Input: part model. Units: mm. Frame: model coordinates. Face numbers are marked on the shaded views. Give positions to 0.01 mm unless a question says otherwise; leave off trailing zeros. Answer as CSV lines item,"result".
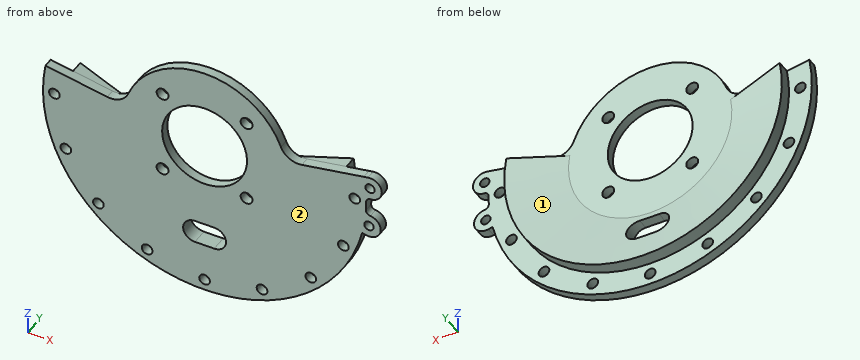
```python
from build123d import *

# Parameters (mm, degrees)
SKETCH1_R           = 1.8
SKETCH1_R_2         = 2
SKETCH1_R_3         = 14.2875
BOSS_EXTRUDE1_DEPTH = 3.175
REVOLVE3_ANGLE      = 200
BOSS_EXTRUDE2_START = -3.175
SKETCH3_R           = 1.5875
BOSS_EXTRUDE2_DEPTH = 3.175
CUT_EXTRUDE1_DEPTH  = 81.857095427


# Read off the part's stored shape, not the designer's step: Revolve3
with BuildPart() as part:
    # Sketch1 → Boss-Extrude1 (new body)
    with BuildSketch(Plane(origin=(0, 0, 0), x_dir=(1, 0, 0), z_dir=(0, 1, 0))):
        with BuildLine():
            Line((53.576531883, -9.446988104), (32.743932203, -5.773638702))
            ThreePointArc((32.743932203, -5.773638702), (28.505328465, -6.505538278), (25.705607757, -9.770963609))
            ThreePointArc((25.705607757, -9.770963609), (0, -27.5), (-25.705607757, -9.770963609))
            ThreePointArc((-25.705607757, -9.770963609), (-28.505328465, -6.505538278), (-32.743932203, -5.773638702))
            Line((-32.743932203, -5.773638702), (-53.576531883, -9.446988104))
            ThreePointArc((-53.576531883, -9.446988104), (0, 54.403036246), (53.576531883, -9.446988104))
        make_face()
        with Locations(Location((-50.569518123, 0, 0), (0, 0, 270))):
            Circle(SKETCH1_R, mode=Mode.SUBTRACT)
        with Locations(Location((-46.720142763, 19.352116768, 0), (0, 0, 270))):
            Circle(SKETCH1_R, mode=Mode.SUBTRACT)
        with Locations(Location((-35.758049186, 35.758049186, 0), (0, 0, 270))):
            Circle(SKETCH1_R, mode=Mode.SUBTRACT)
        with Locations(Location((-19.352116768, 46.720142763, 0), (0, 0, 270))):
            Circle(SKETCH1_R, mode=Mode.SUBTRACT)
        with Locations(Location((0, 50.569518123, 0), (0, 0, 270))):
            Circle(SKETCH1_R, mode=Mode.SUBTRACT)
        with Locations(Location((19.352116768, 46.720142763, 0), (0, 0, 270))):
            Circle(SKETCH1_R, mode=Mode.SUBTRACT)
        with Locations(Location((35.758049186, 35.758049186, 0), (0, 0, 270))):
            Circle(SKETCH1_R, mode=Mode.SUBTRACT)
        with Locations(Location((46.720142763, 19.352116768, 0), (0, 0, 270))):
            Circle(SKETCH1_R, mode=Mode.SUBTRACT)
        with Locations(Location((50.569518123, 0, 0), (0, 0, 270))):
            Circle(SKETCH1_R, mode=Mode.SUBTRACT)
        with Locations(Location((14.142135624, 14.142135624, 0), (0, 0, 270))):
            Circle(SKETCH1_R_2, mode=Mode.SUBTRACT)
        with Locations(Location((-14.142135624, 14.142135624, 0), (0, 0, 270))):
            Circle(SKETCH1_R_2, mode=Mode.SUBTRACT)
        with Locations(Location((-14.142135624, -14.142135624, 0), (0, 0, 270))):
            Circle(SKETCH1_R_2, mode=Mode.SUBTRACT)
        with Locations(Location((14.142135624, -14.142135624, 0), (0, 0, 270))):
            Circle(SKETCH1_R_2, mode=Mode.SUBTRACT)
        with Locations(Location((0, 0, 0), (0, 0, 270))):
            Circle(SKETCH1_R_3, mode=Mode.SUBTRACT)
        with BuildLine():
            Line((-3.25, 37.54875), (3.25, 37.54875))
            ThreePointArc((3.25, 37.54875), (7.21875, 33.58), (3.25, 29.61125))
            Line((3.25, 29.61125), (-3.25, 29.61125))
            ThreePointArc((-3.25, 29.61125), (-7.21875, 33.58), (-3.25, 37.54875))
        make_face(mode=Mode.SUBTRACT)
    extrude(amount=-BOSS_EXTRUDE1_DEPTH)

    # Revolve3 outline → Revolve3 (revolve)
    with BuildSketch(Plane(origin=(0, 0, 0), x_dir=(0.9848077530122042, 0, 0.1736481776669518), z_dir=(-0.1736481776669518, 0, 0.9848077530122042))):
        Polygon((46.736, 0), (46.736, 4.35512275), (27.5, 0), align=None)
    revolve(axis=Axis((0, 0, 0), (0, 1, 0)), revolution_arc=REVOLVE3_ANGLE)

    # Sketch3 → Boss-Extrude2 (add)
    with BuildSketch(Plane.XZ.offset(3.175).offset(BOSS_EXTRUDE2_START)):
        with BuildLine():
            Line((53.060117126, -12.013089669), (54.471072105, -12.3325373))
            ThreePointArc((54.471072105, -12.3325373), (59.259341774, -9.131069871), (55.807809409, -4.519796246))
            ThreePointArc((55.807809409, -4.519796246), (54.72616849, -3.989558211), (54.328198384, -2.85258009))
            ThreePointArc((54.328198384, -2.85258009), (54.387291369, -1.308774374), (54.402523984, 0.236086798))
            ThreePointArc((54.402523984, 0.236086798), (54.854722203, 1.352606489), (55.960615645, 1.830203754))
            ThreePointArc((55.960615645, 1.830203754), (59.629955631, 6.270120891), (55.001219172, 9.698198912))
            Line((55.001219172, 9.698198912), (53.576531883, 9.446988104))
            Line((53.576531883, 9.446988104), (53.060117126, -12.013089669))
        make_face()
        with Locations(Location((55.690385377, 5.789743142, 0), (0, 0, 270))):
            Circle(SKETCH3_R, mode=Mode.SUBTRACT)
        with Locations(Location((55.347437708, -8.461754447, 0), (0, 0, 270))):
            Circle(SKETCH3_R, mode=Mode.SUBTRACT)
    extrude(amount=BOSS_EXTRUDE2_DEPTH)

    # Sketch4 → Cut-Extrude1 (cut, through all)
    with BuildSketch(Plane.XZ):
        with BuildLine():
            Line((-3.25, -37.54875), (3.25, -37.54875))
            ThreePointArc((3.25, -37.54875), (7.21875, -33.58), (3.25, -29.61125))
            Line((3.25, -29.61125), (-3.25, -29.61125))
            ThreePointArc((-3.25, -29.61125), (-7.21875, -33.58), (-3.25, -37.54875))
        make_face()
    extrude(amount=-CUT_EXTRUDE1_DEPTH, mode=Mode.SUBTRACT)


solid = part.part
```
Item 1: Ray query, line 1 (X direction, y = -1.15, z = 0); line 2 (Z direction, x = 13, y = -2); line 3 (Z direction, x = 5, y = -1.5). Return the intervals inside material, ascending. Write a range as from..to.
The answers:
line 1,"-54.4..-52.37, -48.77..-14.29, 14.29..48.77, 52.37..54.4"
line 2,"-52.83..-15.78, -12.5..-5.93, 5.93..12.5, 15.78..24.23"
line 3,"-54.17..-37.14, -30.02..-13.38, 13.38..27.04"
Item 2: Mould query, pull axis X, two halves, no side actions, for the marked faces 1 and 2. Classes: +X half, -X half, draft (parallel to the pull), parting line (faces both ways), or undercut.
The answers:
face 1,"undercut"
face 2,"draft"
Item 3: Contact query for flat-ended pins moving along their axis: pin 1 (6 mm diameter, centred on x = -35.76, z = -35.76, fed in from +Y); pin 2 (3 mm diameter, centred on x = 55.69, z = 5.79, fed in from -Y) (3 decimals); pin 3 (3 mm diameter, centred on x = 1, y = -1, fed in from -Z); pin 4 (2 mm diameter, centred on x = 37, y = 0, fed in from -Z). Output: stop coordinate, or through.
The answers:
pin 1,"y = 0"
pin 2,"through"
pin 3,"z = -54.4"
pin 4,"z = -40.79"
Item 4: Cut plane A-A on y = -1.5. Count the separate pieces of the cut face and the enclosed holes in it, plus the area to 3 significant figures.
The answers:
separate pieces,"1"
enclosed holes,"17"
area,"5,410 mm²"
